Geometry check sheet. Reference: the model listing, model coordinates, mm. A direction names the side the tool comes from. Round coordinates to 2 decimals unless told otherwise and drop trailing zeros. Order: outer loops, then holes, each group sorted by start corner. A loop starts at its lowest first (then second) coordinate and runs counter-clockwise, first axis right, second up.
Autodesk Inventor part; units mm, degrees
ref_plane "YZ Plane" through (0, 0, 0) normal (1, 0, 0) x (0, 1, 0)
ref_plane "XZ Plane" through (0, 0, 0) normal (0, 1, 0) x (-1, 0, 0)
ref_plane "XY Plane" through (0, 0, 0) normal (0, 0, 1) x (1, 0, 0)
sketch "Sketch2" plane through (0, 0, 0) normal (0, 1, 0) x (-1, 0, 0)
  line L0 (0, 0) -> (31.75, 0)
  line L1 (31.75, 0) -> (31.75, -31.75)
  line L2 (31.75, -31.75) -> (0, -31.75)
  line L3 (0, -31.75) -> (0, 0)
  dimension "d0" = 31.75
  dimension "d1" = 31.75
extrude "Extrusion1" add sketch "Sketch2" along normal blind 31.75
sketch "Sketch3" plane through (-31.75, 0, 0) normal (0, 0, 1) x (1, 0, 0)
  line L0 (0, 31.75) -> (31.75, 31.75)
  line L1 (28.575, 31.75) -> (0, 3.175)
  line L2 (0, 0) -> (0, 31.75)
  line L3 (28.575, 31.75) -> (68.9862, 31.75) construction
  line L4 (0, 0) -> (0, 31.75)
  line L5 (0, 31.75) -> (14.2875, 17.4625) construction
  point P0 (31.75, 0)
  dimension "d4" = 135
  dimension "d25" = 3.175
  dimension "d26" = 20.2056
extrude "Extrusion2" cut sketch "Sketch3" against normal blind 38.1
sketch "Sketch4" plane through (0, 0, 0) normal (0, -1, 0) x (1, 0, 0)
  line L0 (-31.75, 0) -> (0, -31.75) construction
  circle A0 centre (-15.875, -15.875) radius 11.0808
  point P0 (0, 0)
  dimension "d7" = 22.1615
extrude "Extrusion3" add sketch "Sketch4" along normal blind 31.75
sketch "Sketch5" plane through (-15.875, -31.75, -15.875) normal (0, -1, 0) x (1, 0, 0)
  circle A0 centre (0, 0) radius 8.7313
  circle A1 centre (0, 0) radius 11.0808
  point P0 (15.875, 15.875)
  dimension "d35" = 17.4625
extrude "Extrusion4" cut sketch "Sketch5" against normal through all contours A0
sketch "Sketch6" plane through (0, 0, 0) normal (1, 0, 0) x (0, 0, -1)
  line L0 (0, 31.75) -> (31.75, 0) construction
  line L1 (4.2545, 4.2545) -> (27.4955, 4.2545) construction
  line L2 (27.4955, 4.2545) -> (27.4955, 27.4955) construction
  line L3 (27.4955, 27.4955) -> (4.2545, 27.4955) construction
  line L4 (4.2545, 27.4955) -> (4.2545, 4.2545) construction
  line L5 (4.2545, 4.2545) -> (27.4955, 27.4955) construction
  line L6 (27.4955, 4.2545) -> (4.2545, 27.4955) construction
  circle A0 centre (4.2545, 27.4955) radius 1.5
  circle A1 centre (4.2545, 4.2545) radius 1.5
  circle A2 centre (27.4955, 4.2545) radius 1.5
  circle A3 centre (27.4955, 27.4955) radius 1.5
  line L7 (0, 31.75) -> (31.75, 31.75)
  point P0 (0, 0)
  point P1 (15.875, 15.875)
  dimension "d15" = 23.241
  dimension "d16" = 23.241
  dimension "d17" = 3
  dimension "d20" = 360
  dimension "d24" = 4.2545
extrude "Extrusion5" cut sketch "Sketch6" against normal blind 12.7
thread "Thread1"
thread "Thread2"
thread "Thread3"
thread "Thread4"
properties part number "motormount" material "Aluminum 6061"
(1) Sectioned sample at A-A, the plane x = -21.5. Record the cut outline in (y, z) (3 decimals), and give its area (3 significant figures).
Returned:
outline: (-31.75, -25.422) - (0, -25.422) - (0, -31.75) - (13.425, -31.75) - (13.425, -22.553) - (-31.75, -22.553) - close; (-31.75, -9.197) - (13.425, -9.197) - (13.425, 0) - (0, 0) - (0, -6.328) - (-31.75, -6.328) - close
area: 429 mm2
(2) Sectioned sample at D-D, the plane y = 16. Record the cut outline in (x, z) (3 decimals).
Returned:
outline: (-18.925, -31.75) - (0, -31.75) - (0, 0) - (-18.925, 0) - (-18.925, -7.694) arc R8.731 cw (long way) to (-18.925, -24.056) - close
(3) Material ranges on line 1 (Z direction, x = -12, y = 2); line 2 (Z direction, x = -2, y = 5); line 3 (Z direction, x = -23.5, y = 5), recorded low to high.
Returned:
line 1: z = -31.75 to -23.7, -8.05 to 0
line 2: z = -31.75 to -28.8, -26.19 to -5.56, -2.95 to 0
line 3: z = -31.75 to -20.13, -11.62 to 0
(4) Sectioned sample at C-C, the plane x = -12. Give the number of separate pieces and of enclosed holes in the cut face, and give its area (3 significant figures).
Returned:
separate pieces: 2
enclosed holes: 2
area: 517 mm2
(5) Set-up check for faces 1 (the flat face through (0, 16, -16)), 2 (the flat face through (-12.7, 4, -27)), 3 (the cylindrical face through (-9.92, -15.65, -25.22)): record each of +Z, -Z, +X, -X, +Y, -Y from which the full face is reachable in a straight line by a thin tool's end or side.
Returned:
face 1: +Z, -Z, +X, +Y, -Y
face 2: +X
face 3: -Y
(6) Sectioned sample at B-B, the plane z = -18.5. Record the cut outline in (x, y) (3 decimals), and give its area (3 significant figures).
Returned:
outline: (-31.75, 0) - (-26.64, 0) - (-26.64, -31.75) - (-24.202, -31.75) - (-24.202, 10.723) - (-31.75, 3.175) - close; (-7.548, -31.75) - (-5.11, -31.75) - (-5.11, 0) - (0, 0) - (0, 31.75) - (-3.175, 31.75) - (-7.548, 27.377) - close
area: 437 mm2
(7) Draft check along Y on faces 4 (the flat face through (-5, 0, -12)), 5 (the flat face through (-17.262, 17.663, -5.069)), 6 (the cylindrical face through (-6.26, 5.74, -4.06)). Enter one of: released by +Y, released by -Y, zero draft, split by the parting line, or undercut.
Returned:
face 4: released by -Y
face 5: released by +Y
face 6: undercut
(8) Depth check by flat-ended pin: P1, Ø1.5, axis at y = -12.5, z = -7, coming from the +X side; P2, Ø2.5, axis at y = 27.5, z = -27.5, coming from the -X side; P3, Ø1.5, axis at x = -6.5, y = -1, coming from the +Z side; P4, Ø1.5, axis at x = -15.5, y = -5, coming from the -Z side. Enter the tip coordinate at first touch or a pass-through.
Returned:
P1: stops at x = -8.34
P2: passes through
P3: stops at z = -8.92
P4: stops at z = -26.96
